For this review, take the finished solid that the model builds, in its own axes (mm). A direction names the side the tool comes from. Coordinates: 2 decimals unless noted, no trailing zeros. Write each loop counter-clockwise with the first axis right and the second up, starting at its lowest first coordinate (ties: lowest second). Pieces come first, ordered by that corner, then holes. Notation, with made-up numbers: (-8, 77.5) -> (8, 77.5) arc R24 ccw to (8, 104.5) -> close; hole circle Ø4 at (77, -11). An arc over 180 degrees is marked (long way). Put each result on its own line as item: value. Start each with the question number.
Item 1: For faces 1 (the cylindrical face through (15.447, 4.014, -34.883)), 2 (the cylindrical face through (17.882, 1.479, -37.762)), 3 (the flat face through (53.298, 3.274, -22.314)), list the 3-axis set-ups (+Z, -Z, +X, -X, +Y, -Y) from which the entire face can be reached by the end or side of a thin tool; tool diameter is ignored.
Item 2: The part is to be moulded in two halves that separate along Z. For faces 4 (the flat face through (48, 2, -40)), 5 (the flat face through (53.34, 3.27, -27.51)), 6 (the flat face through (60, 2, -20)), say which applies: +Z half, -Z half, draft (parallel to the pull), parting line (faces both ways), or undercut.
Item 3: Insertion check: P1, Ø7, axis at x = 16.53, z = -6.53, coming from the -Y side. The pin has a flat end and moves straight along its axis. Give the tip position at first contact, or say it passes through.
Item 4: To check wall thickness, follow L1, parallel to X at y = 4.4, z = -33.47 (3 decimals); L2, parallel to Z at x = 8, y = 3.95; L3, parallel to X at y = 0.85, z = -4. State the ranges of each line that lie inside material, in increasing order.
Item 5: Consider section B-B on x = 19.5. Give the boundary of the cut face in (y, z), and give its area (3 significant figures).
Item 6: Consider section D-D on x = 42.5. Give the boundary of the cut face in (y, z), and give its area (3 significant figures).
Item 7: Consider section C-C on z = -27.5. Give the boundary of the cut face in (x, y), and give its area (3 significant figures).
Item 8: Consider section A-A on z = -16. Give the boundary of the cut face in (x, y).
```python
from build123d import *

# Parameters (mm, degrees)
SKETCH1_W           = 60
SKETCH1_H           = 40
BOSS_EXTRUDE1_DEPTH = 5
SKETCH2_R           = 1.78
SKETCH2_R_2         = 1.905
CUT_EXTRUDE1_DEPTH  = 10
CUT_EXTRUDE2_DEPTH  = 73.284161474
SKETCH7_R           = 4.5
CUT_EXTRUDE5_DEPTH  = 3
CUT_EXTRUDE6_DEPTH  = 3.5


with BuildPart() as part:
    # Sketch1 → Boss-Extrude1 (new body)
    with BuildSketch(Plane(origin=(0, 0, 0), x_dir=(1, 0, 0), z_dir=(0, 1, 0))):
        with Locations((30, 20)):
            Rectangle(SKETCH1_W, SKETCH1_H)
    extrude(amount=BOSS_EXTRUDE1_DEPTH)

    # Sketch2 → Cut-Extrude1 (cut)
    with BuildSketch(Plane(origin=(0, 5, 0), x_dir=(1, 0, 0), z_dir=(0, 1, 0))):
        with Locations(Location((43.47, 33.47, 0), (0, 0, 270))):
            Circle(SKETCH2_R)
        with Locations(Location((16.53, 33.47, 0), (0, 0, 270))):
            Circle(SKETCH2_R)
        with Locations(Location((16.53, 6.53, 0), (0, 0, 270))):
            Circle(SKETCH2_R)
        with Locations(Location((43.47, 6.53, 0), (0, 0, 270))):
            Circle(SKETCH2_R)
        with Locations(Location((54.818710608, 24.9, 0), (0, 0, 270))):
            Circle(SKETCH2_R_2)
        with Locations(Location((5.288710608, 24.9, 0), (0, 0, 270))):
            Circle(SKETCH2_R_2)
        with Locations(Location((5.288710608, 15.1, 0), (0, 0, 270))):
            Circle(SKETCH2_R_2)
        with Locations(Location((54.818710608, 15.1, 0), (0, 0, 270))):
            Circle(SKETCH2_R_2)
    extrude(amount=-CUT_EXTRUDE1_DEPTH, mode=Mode.SUBTRACT)

    # Sketch3 → Cut-Extrude2 (cut, through all)
    with BuildSketch(Plane(origin=(0, 5, 0), x_dir=(1, 0, 0), z_dir=(0, 1, 0))):
        with BuildLine():
            ThreePointArc((36.230094697, 31.976473607), (33.206836939, 33.113588252), (30, 33.5))
            Line((30, 33.5), (30, 27.34780867))
            Line((30, 27.34780867), (36.230094697, 27.34780867))
            Line((36.230094697, 27.34780867), (36.230094697, 31.976473607))
        make_face()
        with BuildLine():
            Line((36.230094697, 27.34780867), (30, 27.34780867))
            Line((30, 27.34780867), (30, 6.5))
            ThreePointArc((30, 6.5), (39.545941546, 10.454058454), (43.5, 20))
            ThreePointArc((43.5, 20), (41.540283324, 27.005131033), (36.230094697, 31.976473607))
            Line((36.230094697, 31.976473607), (36.230094697, 27.34780867))
        make_face()
        with BuildLine():
            Line((30, 27.34780867), (30, 33.5))
            ThreePointArc((30, 33.5), (27.414652789, 33.250131312), (24.925008883, 32.509774785))
            Line((24.925008883, 32.509774785), (24.925008883, 27.34780867))
            Line((24.925008883, 27.34780867), (30, 27.34780867))
        make_face()
        with BuildLine():
            Line((30, 6.5), (30, 27.34780867))
            Line((30, 27.34780867), (24.925008883, 27.34780867))
            Line((24.925008883, 27.34780867), (24.925008883, 32.509774785))
            ThreePointArc((24.925008883, 32.509774785), (16.749868688, 17.414652789), (30, 6.5))
        make_face()
        with BuildLine():
            Line((36.230094697, 40), (30, 40))
            Line((30, 40), (30, 33.5))
            ThreePointArc((30, 33.5), (33.206836939, 33.113588252), (36.230094697, 31.976473607))
            Line((36.230094697, 31.976473607), (36.230094697, 40))
        make_face()
        with BuildLine():
            Line((30, 33.5), (30, 40))
            Line((30, 40), (24.925008883, 40))
            Line((24.925008883, 40), (24.925008883, 32.509774785))
            ThreePointArc((24.925008883, 32.509774785), (27.414652789, 33.250131312), (30, 33.5))
        make_face()
    extrude(amount=-CUT_EXTRUDE2_DEPTH, mode=Mode.SUBTRACT)

    # Sketch7 → Cut-Extrude5 (cut)
    with BuildSketch(Plane(origin=(0, 0, 0), x_dir=(-1, 0, 0), z_dir=(0, -1, 0))):
        with Locations(Location((-43.47, 6.53, 0), (0, 0, 90))):
            Circle(SKETCH7_R)
        with Locations(Location((-16.53, 6.53, 0), (0, 0, 90))):
            Circle(SKETCH7_R)
        with Locations(Location((-16.53, 33.47, 0), (0, 0, 90))):
            Circle(SKETCH7_R)
        with Locations(Location((-43.47, 33.47, 0), (0, 0, 90))):
            Circle(SKETCH7_R)
    extrude(amount=-CUT_EXTRUDE5_DEPTH, mode=Mode.SUBTRACT)

    # Sketch8 → Cut-Extrude6 (cut)
    with BuildSketch(Plane(origin=(0, 5, 0), x_dir=(1, 0, 0), z_dir=(0, 1, 0))):
        Polygon((5.288710608, 18.564101615), (2.288710608, 16.832050808), (2.288710608, 13.367949192), (5.288710608, 11.635898385), (8.288710608, 13.367949192), (8.288710608, 16.832050808), align=None)
        Polygon((54.818710608, 11.635898385), (57.818710608, 13.367949192), (57.818710608, 16.832050808), (54.818710608, 18.564101615), (51.818710608, 16.832050808), (51.818710608, 13.367949192), align=None)
        Polygon((5.288710608, 28.364101615), (2.288710608, 26.632050808), (2.288710608, 23.167949192), (5.288710608, 21.435898385), (8.288710608, 23.167949192), (8.288710608, 26.632050808), align=None)
        Polygon((54.818710608, 28.364101615), (51.818710608, 26.632050808), (51.818710608, 23.167949192), (54.818710608, 21.435898385), (57.818710608, 23.167949192), (57.818710608, 26.632050808), align=None)
    extrude(amount=-CUT_EXTRUDE6_DEPTH, mode=Mode.SUBTRACT)


solid = part.part
```
Return value:
1. face 1: +Y, -Y
1. face 2: -Y
1. face 3: +Y
2. face 4: -Z half
2. face 5: undercut
2. face 6: draft
3. P1: y = 3
4. L1: 0 to 14.75, 18.31 to 24.925, 36.23 to 41.69, 45.25 to 60
4. L2: -40 to -26.8, -23 to -17, -13.2 to 0
4. L3: 0 to 12.81, 20.25 to 39.75, 47.19 to 60
5. outline: (0, -40) -> (5, -40) -> (5, -28.49) -> (0, -28.49) -> (0, -30.09) -> (3, -30.09) -> (3, -36.85) -> (0, -36.85) -> close; (0, -11.51) -> (5, -11.51) -> (5, 0) -> (0, 0) -> (0, -3.15) -> (3, -3.15) -> (3, -9.91) -> (0, -9.91) -> close
5. area: 74.6 mm^2
6. outline: (0, -40) -> (5, -40) -> (5, -34.96) -> (3, -34.96) -> (3, -37.86) -> (0, -37.86) -> close; (0, -29.08) -> (3, -29.08) -> (3, -31.98) -> (5, -31.98) -> (5, -25.1) -> (0, -25.1) -> close; (0, -14.9) -> (5, -14.9) -> (5, -8.02) -> (3, -8.02) -> (3, -10.92) -> (0, -10.92) -> close; (0, -2.14) -> (3, -2.14) -> (3, -5.04) -> (5, -5.04) -> (5, 0) -> (0, 0) -> close
6. area: 84.3 mm^2
7. outline: (0, 0) -> (18.78, 0) -> (18.78, 5) -> (6.79, 5) -> (6.79, 1.5) -> (3.79, 1.5) -> (3.79, 5) -> (0, 5) -> close; (41.22, 0) -> (60, 0) -> (60, 5) -> (56.32, 5) -> (56.32, 1.5) -> (53.32, 1.5) -> (53.32, 5) -> (41.22, 5) -> close
7. area: 167 mm^2
8. outline: (0, 0) -> (3.61, 0) -> (3.61, 1.5) -> (2.29, 1.5) -> (2.29, 5) -> (0, 5) -> close; (6.97, 0) -> (17.11, 0) -> (17.11, 5) -> (8.29, 5) -> (8.29, 1.5) -> (6.97, 1.5) -> close; (42.89, 0) -> (53.14, 0) -> (53.14, 1.5) -> (51.82, 1.5) -> (51.82, 5) -> (42.89, 5) -> close; (56.5, 0) -> (60, 0) -> (60, 5) -> (57.82, 5) -> (57.82, 1.5) -> (56.5, 1.5) -> close
